Could you check a few things on this model? Use its own coordinates, in mm. Coordinates: 2 decimals unless noted, no trailing zeros. Loops run counter-clockwise (first coordinate to the right, second up) from the corner with the lowest first, then second, coordinate; pieces in that order, holes last.
1) Imagine slicing it at D-D on z = -36. Please give me the cut outline in (x, y).
2) Will this pin go through, and if not, where does the flat tip stop? P1, Ø3.5, axis at x = 82.5, z = -36, coming from the +Y side.
3) Imagine slicing it at B-B on z = -21. Please give me the cut outline in (x, y), plus the area to 3 significant figures.
4) Thinking about a two-plate mould opening in Z: for faces 1 (the face through (44, 2, -42)), 2 (the face through (1, 3, -2)), 3 (the face through (0, 2, -21)), 4 (the face through (28.4, 2.46, -21.09)), which applies, released by +Z, released by -Z, zero draft, split by the parting line, or undercut?
5) Imagine slicing it at A-A on x = 59.5. Please give me the cut outline in (y, z).
6) If I drill on line 1 along Z through (x, y) = (7.5, 2.5); line 2 along X through (y, z) = (3.3, -21); line 3 along X through (y, z) = (3.6, -36), over which ranges is the centre line in solid material (lowest first)?
7) Imagine slicing it at C-C on x = 7.5. Please give me the cut outline in (y, z), plus the area to 3 significant figures.
```python
from build123d import *

# Parameters (mm, degrees)
SKETCH1_W           = 90
SKETCH1_H           = 42
SKETCH1_R           = 9.5
SKETCH1_R_2         = 2.1
SKETCH1_R_3         = 1.45
BOSS_EXTRUDE1_DEPTH = 5
FILLET1_R           = 5


with BuildPart() as part:
    # Sketch1 → Boss-Extrude1 (new body)
    with BuildSketch(Plane(origin=(0, 0, 0), x_dir=(1, 0, 0), z_dir=(0, 1, 0))):
        with Locations((45, 21)):
            Rectangle(SKETCH1_W, SKETCH1_H)
        with Locations((45, 21)):
            Circle(SKETCH1_R, mode=Mode.SUBTRACT)
        with Locations((59.5, 21)):
            Circle(SKETCH1_R_2, mode=Mode.SUBTRACT)
        with Locations((30.5, 21)):
            Circle(SKETCH1_R_2, mode=Mode.SUBTRACT)
        with Locations((7.5, 36)):
            Circle(SKETCH1_R_3, mode=Mode.SUBTRACT)
        with Locations((7.5, 6)):
            Circle(SKETCH1_R_3, mode=Mode.SUBTRACT)
        with Locations((82.5, 6)):
            Circle(SKETCH1_R_3, mode=Mode.SUBTRACT)
        with Locations((82.5, 36)):
            Circle(SKETCH1_R_3, mode=Mode.SUBTRACT)
    extrude(amount=BOSS_EXTRUDE1_DEPTH)

    # Fillet1
    fillet1_edges = [part.edges().sort_by_distance(p)[0] for p in [
        (0, 2.5, -42),
        (90, 2.5, -42),
        (90, 2.5, 0),
        (0, 2.5, 0),
    ]]
    fillet(fillet1_edges, radius=FILLET1_R)


solid = part.part
```
Filled in:
1. outline: (0, 0) - (6.05, 0) - (6.05, 5) - (0, 5) - close; (8.95, 0) - (81.05, 0) - (81.05, 5) - (8.95, 5) - close; (83.95, 0) - (90, 0) - (90, 5) - (83.95, 5) - close
2. P1: stops at y = 5
3. outline: (0, 0) - (28.4, 0) - (28.4, 5) - (0, 5) - close; (32.6, 0) - (35.5, 0) - (35.5, 5) - (32.6, 5) - close; (54.5, 0) - (57.4, 0) - (57.4, 5) - (54.5, 5) - close; (61.6, 0) - (90, 0) - (90, 5) - (61.6, 5) - close
3. area: 313 mm2
4. face 1: released by -Z
4. face 2: released by +Z
4. face 3: zero draft
4. face 4: undercut
5. outline: (0, -42) - (5, -42) - (5, -23.1) - (0, -23.1) - close; (0, -18.9) - (5, -18.9) - (5, 0) - (0, 0) - close
6. line 1: z = -42 to -37.45, -34.55 to -7.45, -4.55 to 0
6. line 2: x = 0 to 28.4, 32.6 to 35.5, 54.5 to 57.4, 61.6 to 90
6. line 3: x = 0 to 6.05, 8.95 to 81.05, 83.95 to 90
7. outline: (0, -42) - (5, -42) - (5, -37.45) - (0, -37.45) - close; (0, -34.55) - (5, -34.55) - (5, -7.45) - (0, -7.45) - close; (0, -4.55) - (5, -4.55) - (5, 0) - (0, 0) - close
7. area: 181 mm2
